The listing builds one solid part. Answer for the finished solid, in the listing's coordinates (mm). A direction names the side the tool comes from. Coordinates: 2 decimals unless noted, no trailing zeros. Answer in a Markdown table with one row per item. Add a question column.
Autodesk Inventor part; units mm, degrees
ref_plane "YZ Plane" through (0, 0, 0) normal (1, 0, 0) x (0, 1, 0)
ref_plane "XZ Plane" through (0, 0, 0) normal (0, 1, 0) x (-1, 0, 0)
ref_plane "XY Plane" through (0, 0, 0) normal (0, 0, 1) x (1, 0, 0)
sketch "Sketch1" plane through (0, 0, 0) normal (0, 1, 0) x (-1, 0, 0)
  circle A0 centre (0, 0) radius 50.8
  dimension "d0" = 101.6
extrude "Extrusion1" add sketch "Sketch1" along normal blind 7.62
sketch "Sketch2" plane through (0, 7.62, 0) normal (0, 1, 0) x (1, 0, 0)
  circle A0 centre (0, 0) radius 49.2125
  circle A1 centre (0, 0) radius 50.8
  dimension "d3" = 98.425
extrude "Extrusion2" cut sketch "Sketch2" against normal blind 3.175
sketch "Sketch3" plane through (0, 7.62, 0) normal (0, 1, 0) x (1, 0, 0)
  circle A0 centre (0, 0) radius 50.9584
extrude "Extrusion3" add sketch "Sketch3" along normal blind 7.62
sketch "Sketch4" plane through (0, 15.24, 0) normal (0, 1, 0) x (1, 0, 0)
  point P0 (0, 0)
sketch "Sketch5" plane through (0, 15.24, 0) normal (0, 1, 0) x (1, 0, 0)
  circle A0 centre (0, 0) radius 49.2125
  circle A1 centre (0, 0) radius 50.9584
  dimension "d8" = 98.425
extrude "Extrusion4" cut sketch "Sketch5" against normal blind 3.175
sketch "Sketch6" plane through (0, 15.24, 0) normal (0, 1, 0) x (1, 0, 0)
  circle A0 centre (0, 0) radius 50.8
  dimension "d11" = 101.6
extrude "Extrusion5" add sketch "Sketch6" along normal blind 5.08
sketch "Sketch7" plane through (0, 0, 0) normal (0, -1, 0) x (1, 0, 0)
  circle A0 centre (0, 0) radius 57.15
  dimension "d14" = 114.3
extrude "Extrusion6" add sketch "Sketch7" along normal blind 6.096
chamfer "Chamfer1" distance 2.54 angle 45 1 edges at (-50.8, 20.32, 0)
sketch "Sketch8" plane through (0, -6.096, 0) normal (0, -1, 0) x (1, 0, 0)
  circle A0 centre (0, 0) radius 50.8
  circle A1 centre (53.975, 0) radius 1.7526
  circle A2 centre (26.9875, 46.7437) radius 1.7526
  circle A3 centre (-26.9875, 46.7437) radius 1.7526
  circle A4 centre (-53.975, 0) radius 1.7526
  circle A5 centre (-26.9875, -46.7437) radius 1.7526
  circle A6 centre (26.9875, -46.7437) radius 1.7526
  dimension "d20" = 3.5052
  dimension "d21" = 53.975
  dimension "d24" = 360
extrude "Extrusion7" cut sketch "Sketch8" against normal blind 6.096 contours A1 | A2 | A3 | A4 | A5 | A6
sketch "Sketch9" plane through (0, -6.096, 0) normal (0, -1, 0) x (1, 0, 0)
  circle A0 centre (0, 0) radius 12.7
  circle A1 centre (0, 0) radius 1.27
  dimension "d28" = 25.4
  dimension "d29" = 2.54
extrude "Extrusion8" cut sketch "Sketch9" against normal blind 127 contours A1
sketch "Sketch10" plane through (0, -6.096, 0) normal (0, -1, 0) x (1, 0, 0)
  circle A0 centre (0, 0) radius 1.27
  circle A1 centre (0, 0) radius 38.1
  dimension "d33" = 76.2
extrude "Extrusion9" cut sketch "Sketch10" against normal blind 9.525
sketch "Sketch11" plane through (0, 3.429, 0) normal (0, -1, 0) x (1, 0, 0)
  circle A0 centre (0, 0) radius 12.7
  circle A1 centre (0, 0) radius 1.27
  dimension "d36" = 25.4
extrude "Extrusion10" add sketch "Sketch11" along normal blind 9.525
properties part number "O ring Plug 1"
(1) The mould has two halves that part along Z. Classify faces 4 (the face through (-2.75, -1.27, 12.4)), 5 (the face through (-27, 4.445, -42)), 6 (the face through (46.94, 6.05, -14.78)): released by +Z, released by -Z, zero draft, split by the parting line, or undercut.
(2) For faces 1 (the face through (16, 3.429, 1)), 2 (the face through (-27, 15.24, -42)), 3 (the face through (48.605, 9.811, 15.307)), determine the directions among +Z, -Z, +X, -X, +Y, -Y from which every point of the face is accessible in a straight line to the end or side of a thin tool.
(3) A cutting plane is placed at A-A (y = -3.5). State how many separate pieces and enclosed holes the cut face has, plus the area to 3 significant figures.
(4) Straight lines are drawn through the part: line 1 (Z direction, x = 0, y = 4.75); line 2 (Z direction, x = 6.5, y = -0.5); line 3 (Y direction, x = -23, z = 45.5). For each, find the intervals that lie inside material, in ascending order.
(5) Each of these flat-tipped pins is pushed along its axis until it touches: pin 1 (5 mm diameter, centred on x = -38.5, y = 10, fed in from -Z); pin 2 (3 mm diameter, centred on x = -26.99, z = 46.74, fed in from +Y); pin 3 (2 mm diameter, centred on y = 16.5, z = 28, fed in from -X); pin 4 (10 mm diameter, centred on y = 7.5, z = -2, fed in from -X). Where does it stop, or does it pass through?
Solved:
| question | item | result |
|---|---|---|
| 1 | face 4 | undercut |
| 1 | face 5 | zero draft |
| 1 | face 6 | split by the parting line |
| 2 | face 1 | -Y |
| 2 | face 2 | none |
| 2 | face 3 | +Y |
| 3 | separate pieces | 2 |
| 3 | enclosed holes | 8 |
| 3 | area | 6,140 mm² |
| 4 | line 1 | z = -49.21 to -1.27, 1.27 to 49.21 |
| 4 | line 2 | z = -56.78 to -37.54, -10.91 to 10.91, 37.54 to 56.78 |
| 4 | line 3 | y = -6.1 to 0 |
| 5 | pin 1 | stops at z = -36.07 |
| 5 | pin 2 | passes through |
| 5 | pin 3 | stops at x = -43.03 |
| 5 | pin 4 | stops at x = -50.96 |
